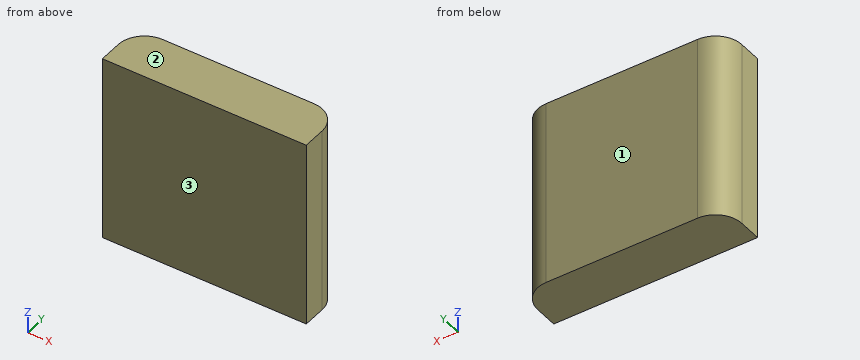
from build123d import *

# Parameters (mm, degrees)
SKETCH1_W           = 62
SKETCH1_H           = 57
BOSS_EXTRUDE1_DEPTH = 15
FILLET1_R           = 8


with BuildPart() as part:
    # Sketch1 → Boss-Extrude1 (new body)
    with BuildSketch(Plane(origin=(0, 0, 0), x_dir=(1, 0, 0), z_dir=(0, 1, 0))):
        with Locations((31, 28.5)):
            Rectangle(SKETCH1_W, SKETCH1_H)
    extrude(amount=BOSS_EXTRUDE1_DEPTH)

    # Fillet1
    fillet1_edges = [part.edges().sort_by_distance(p)[0] for p in [
        (62, 15, -28.5),
        (0, 15, -28.5),
    ]]
    fillet(fillet1_edges, radius=FILLET1_R)


solid = part.part
CAD build for the part. Positions are in the model's coordinates, mm. Face numbers are marked on the shaded views. Give positions to 0.01 mm unless a question says otherwise; leave off trailing zeros. Write each loop counter-clockwise with the first axis right and the second up, starting at its lowest first coordinate (ties: lowest second). Pieces come first, ordered by that corner, then holes. Notation, with made-up numbers: (31, 11.25) - (44, 11.25) arc R14 ccw to (44, 34.25) - close; hole circle Ø4 at (15, 64). An arc over 180 degrees is marked (long way). Put each result on its own line as item: value.
(1) Saw through at B-B (x = 4.5). List the corners of the cut face in (y, z).
Working result:
outline: (0, -57) - (14.19, -57) - (14.19, 0) - (0, 0) - close
(2) Drop flat-ended pins along their axis: pin 1 Ø5 at (y, z) = (12, -16.5) entering from -X; pin 2 Ø5 at (x, z) = (55, -35) entering from -Y; pin 3 Ø3 at (y, z) = (10.5, -28) entering from +X; pin 4 Ø4 at (y, z) = (10.5, -11.5) entering from -X. Give the stop position or say it passes through.
Working result:
pin 1: x = 0.4
pin 2: y = 0
pin 3: x = 61.75
pin 4: x = 0.14
(3) Saw through at C-C (y = 14.25). List the corners of the cut face in (x, z), then the cut area to 3 significant figures.
Working result:
outline: (4.62, -57) - (57.38, -57) - (57.38, 0) - (4.62, 0) - close
area: 3,010 mm^2
(4) Saw through at A-A (z = -5). List the corners of the cut face in (x, y), then the cut area to 3 significant figures.
Working result:
outline: (0, 0) - (62, 0) - (62, 7) arc R8 ccw to (54, 15) - (8, 15) arc R8 ccw to (0, 7) - close
area: 903 mm^2
(5) Wall check: L1, parallel to Y at x = 3.5, z = -42; L2, parallel to X at y = 12.25, z = -42.5; L3, parallel to X at y = 14.25, z = -33. Give the ranges that are in metal, low to high.
Working result:
L1: 0 to 13.61
L2: 1.96 to 60.04
L3: 4.62 to 57.38
(6) Pull direction Y, two halves, no side cores. Call the marked faces 1, 2 and 3: released by +Y, released by -Y, zero draft, split by the parting line, or undercut.
Working result:
face 1: released by +Y
face 2: zero draft
face 3: released by -Y
